Autodesk Inventor part; units mm, degrees
ref_plane "YZ Plane" through (0, 0, 0) normal (1, 0, 0) x (0, 1, 0)
ref_plane "XZ Plane" through (0, 0, 0) normal (0, 1, 0) x (-1, 0, 0)
ref_plane "XY Plane" through (0, 0, 0) normal (0, 0, 1) x (1, 0, 0)
sketch "Sketch1" plane through (0, 0, 0) normal (0, 0, 1) x (1, 0, 0)
  line L0 (0, 0) -> (-32, 0)
  line L1 (-32, 0) -> (-32, 76)
  line L2 (-32, 76) -> (0, 76)
  line L3 (0, 76) -> (0, 0)
  dimension "d0" = 32
  dimension "d1" = 76
extrude "Extrusion1" add sketch "Sketch1" along normal blind 18
fillet "Fillet1" radius 6 4 edges at (0, 76, 9) (-32, 76, 9) (0, 0, 9) (-32, 0, 9)
sketch "Sketch2" plane through (0, 0, 18) normal (0, 0, 1) x (1, 0, 0)
  line L0 (-6, 58) -> (-26, 58)
  line L1 (-26, 58) -> (-26, 18)
  line L2 (-26, 18) -> (-6, 18)
  line L3 (-6, 18) -> (-6, 58)
  line L4 (-6, 76) -> (-26, 76)
  line L5 (0, 6) -> (0, 70)
  point P0 (0, 0)
  dimension "d5" = 20
  dimension "d6" = 40
  dimension "d7" = 18
  dimension "d8" = 6
extrude "Extrusion2" cut sketch "Sketch2" against normal blind 12.5
sketch "Sketch3" plane through (0, 0, 5.5) normal (0, 0, 1) x (1, 0, 0)
  circle A0 centre (-16, 28) radius 6.75
  line L0 (-6, 58) -> (-6, 18)
  line L1 (-6, 18) -> (-26, 18)
  point P0 (0, 0)
  dimension "d11" = 13.5
  dimension "d12" = 10
  dimension "d13" = 10
extrude "Extrusion3" cut sketch "Sketch3" against normal up to surface (5.5 mm away)
sketch "Sketch4" plane through (0, 0, 18) normal (0, 0, 1) x (1, 0, 0)
  line L0 (-26, 58) -> (-6, 58)
  line L1 (-6, 58) -> (-26, 58)
  line L2 (-26, 58) -> (-26, 65.7)
  line L3 (-26, 65.7) -> (-6, 65.7)
  line L4 (-6, 65.7) -> (-6, 58)
  line L5 (-6, 18) -> (-26, 18)
  line L6 (-6, 18) -> (-26, 18)
  line L7 (-26, 18) -> (-26, 10.3)
  line L8 (-26, 10.3) -> (-6, 10.3)
  line L9 (-6, 10.3) -> (-6, 18)
  point P0 (0, 0)
  point P1 (-26, 18)
  dimension "d16" = 7.7
  dimension "d17" = 20
  dimension "d18" = 7.7
extrude "Extrusion4" cut sketch "Sketch4" against normal blind 5
sketch "Sketch5" plane through (0, 6, 0) normal (1, 0, 0) x (0, 0, -1)
  line L0 (0, -6) -> (-18, -6)
  line L1 (0, -6) -> (0, 4)
  line L2 (0, 0) -> (0, -6)
  line L3 (0, 4) -> (-10, 4)
  line L4 (-10, 4) -> (-10, -6)
  line L5 (0, 70) -> (0, 64)
  line L6 (0, 70) -> (-10, 70)
  line L7 (-10, 70) -> (-10, 60)
  line L8 (-10, 60) -> (0, 60)
  line L9 (0, 60) -> (0, 70)
  dimension "d21" = 10
  dimension "d22" = 10
  dimension "d23" = 10
  dimension "d24" = 10
extrude "Extrusion5" cut sketch "Sketch5" against normal up to surface (32 mm away)
fillet "Fillet2" radius 3 20 edges at (-16, 66, 0) (0, 38, 0) (-16, 10, 0) (-32, 38, 0) (0, 66, 5) (-32, 66, 5) (0, 10, 5) (-16, 66, 10) (-32, 10, 5) (-16, 10, 10) (-16, 76, 10) (-30.2426, 74.2426, 10) (-32, 68, 10) (0, 68, 10) (-1.7574, 74.2426, 10) (-1.7574, 1.7574, 10) (0, 8, 10) (-30.2426, 1.7574, 10) (-32, 8, 10) (-16, 0, 10)
sketch "Sketch6" plane through (-3, 69, 10) normal (0, 0, -1) x (-1, 0, 0)
  arc A0 (26, 1) -> (23, 4) centre (23, 1) ccw
  circle A1 centre (23, 1) radius 1.2
  arc A2 (3, 4) -> (0, 1) centre (3, 1) ccw
  circle A3 centre (3, 1) radius 1.2
  arc A4 (0, -63) -> (3, -66) centre (3, -63) ccw
  circle A5 centre (3, -63) radius 1.2
  arc A6 (23, -66) -> (26, -63) centre (23, -63) ccw
  circle A7 centre (23, -63) radius 1.2
  point P0 (-3, -69)
  dimension "d28" = 2.4
  dimension "d29" = 2.4
  dimension "d30" = 2.4
  dimension "d31" = 2.4
extrude "Extrusion6" cut sketch "Sketch6" along normal blind 5 and the other way blind 10
sketch "Sketch7" plane through (0, 0, 0) normal (0, 0, -1) x (-1, 0, 0)
  circle A0 centre (16, 28) radius 6.75
  circle A1 centre (16, 28) radius 11
  point P0 (0, 0)
  dimension "d36" = 22
extrude "Extrusion7" cut sketch "Sketch7" against normal blind 2
fillet "Fillet3" radius 2 1 edges at (-5, 28, 0)
properties part number "ramie03-5"
Input: part model. Units: mm. Frame: model coordinates. A direction names the side the tool comes from. Round coordinates to 2 decimals unless told otherwise and drop trailing zeros. Write each loop counter-clockwise with the first axis right and the second up, starting at its lowest first coordinate (ties: lowest second). Pieces come first, ordered by that corner, then holes. Notation, with made-up numbers: (72.5, 32.25) - (118.5, 32.25) arc R17 cw to (118.5, 37.25) - close; hole circle Ø7 at (54, 70.5). An arc over 180 degrees is marked (long way). Write item = value, one per line.
(1) Section query D-D on z = 11.5. State how many separate pieces and enclosed holes the cut face has, then the cut area to 3 significant figures.
Geometry check:
separate_pieces = 1
enclosed_holes = 5
area = 1,550 mm^2
(2) Pull-direction query (X, two-part tool) for faces 4 (the flat face through (-16, 66, 5)), 5 (the cylindrical face through (-30.196, 74.289, 15.535)), 6 (the flat face through (-16, 62, 13)); classes: +X half, -X half, draft (parallel to the pull), parting line (faces both ways), or undercut.
Geometry check:
face_4 = draft
face_5 = -X half
face_6 = undercut
(3) Material intervals for probe 1 along X at (y, z) = (70, 13.75); probe 2 along X at (y, z) = (28, 5.25); probe 3 along X at (y, z) = (36.5, 15.75), sorted ascending.
Geometry check:
probe_1 = -32 to -27.2, -24.8 to -7.2, -4.8 to 0
probe_2 = -32 to -22.75, -9.25 to 0
probe_3 = -32 to -26, -6 to 0
(4) Access query for faces 1 (the cylindrical face through (-31.14, 10.9, 5.03)), 2 (the cylindrical face through (-31.14, 69.49, 10.9)), 3 (the cylindrical face through (-0.86, 69.51, 10.9)). Directions: +Z, -Z, +X, -X, +Y, -Y. A direction counts if a zero-diameter tool reaches every point of the face in a straight line with its end or side. Return the directions, or none.
Geometry check:
face_1 = -Z, -X, -Y
face_2 = -Z, -X, +Y
face_3 = -Z, +X, +Y
(5) Contact query for flat-ended pins moving along their axis: pin 1 Ø2 at (x, z) = (-13, 9.5) entering from +Y; pin 2 Ø3 at (x, y) = (-18, 31.5) entering from +Z; pin 3 Ø1.2 at (x, y) = (-15.5, 5.5) entering from -Z; pin 4 Ø8 at (x, z) = (-20.5, 8.5) entering from -Y. Output: stop coordinate, or through.
Geometry check:
pin_1 = 74.66
pin_2 = through
pin_3 = 10
pin_4 = 0.04
(6) Section query C-C on z = 4.5. Output: boundary loops of the cut face in (x, y).
Geometry check:
outline = (-32, 13) arc R3 ccw to (-29, 10) - (-3, 10) arc R3 ccw to (0, 13) - (0, 63) arc R3 ccw to (-3, 66) - (-29, 66) arc R3 ccw to (-32, 63) - close; hole circle Ø13.5 at (-16, 28)
